from build123d import *
from build123d.topology import SkipClean

# Parameters (mm, degrees)
SKETCH1_R           = 1.2
BOSS_EXTRUDE1_DEPTH = 2.2
BOSS_EXTRUDE2_START = 2.2
SKETCH2_R           = 1.2
BOSS_EXTRUDE2_DEPTH = 2.2
SKETCH3_R           = 1.2
BOSS_EXTRUDE3_DEPTH = 2.2


with BuildPart() as part:
    # Sketch1 → Boss-Extrude1 (new body)
    with BuildSketch(Plane(origin=(0, 0, 0), x_dir=(1, 0, 0), z_dir=(0, 1, 0))):
        with BuildLine():
            Line((-5.035, 1.393945325), (-5.035, 3.24734466))
            Line((-5.035, 3.24734466), (-2.8, 3.24734466))
            Line((-2.8, 3.24734466), (-2.8, 1.393945325))
            ThreePointArc((-2.8, 1.393945325), (-3.9175, -2.24265534), (-5.035, 1.393945325))
        make_face()
        with Locations(Location((-3.9175, -0.25265534, 0), (0, 0, 270))):
            Circle(SKETCH1_R, mode=Mode.SUBTRACT)
    extrude(amount=BOSS_EXTRUDE1_DEPTH)

    # Sketch2 → Boss-Extrude2 (add)
    with SkipClean():  # the faces are left unmerged after this step: merging them gives an invalid solid
        with BuildSketch(Plane.XZ.offset(BOSS_EXTRUDE2_START)):
            Polygon((-3.9175, -3.24734466), (-0.1675, -3.24734466), (-0.1675, 2.75265534), (-7.6675, 2.75265534), (-7.789861557, -3.24734466), align=None)
            with Locations(Location((-3.9175, 0.25265534, 0), (0, 0, 270))):
                Circle(SKETCH2_R, mode=Mode.SUBTRACT)
        extrude(amount=-BOSS_EXTRUDE2_DEPTH)

    # Sketch3 → Boss-Extrude3 (add)
    with BuildSketch(Plane(origin=(0, 2.2, 0), x_dir=(1, 0, 0), z_dir=(0, 1, 0))):
        Polygon((-7.789861557, 3.24734466), (-5.035, 3.24734466), (-2.8, 3.24734466), (-0.1675, 3.24734466), (-0.1675, -2.75265534), (-7.6675, -2.75265534), align=None)
        with Locations(Location((-3.9175, -0.25265534, 0), (0, 0, 90))):
            Circle(SKETCH3_R, mode=Mode.SUBTRACT)
    extrude(amount=BOSS_EXTRUDE3_DEPTH)


solid = part.part
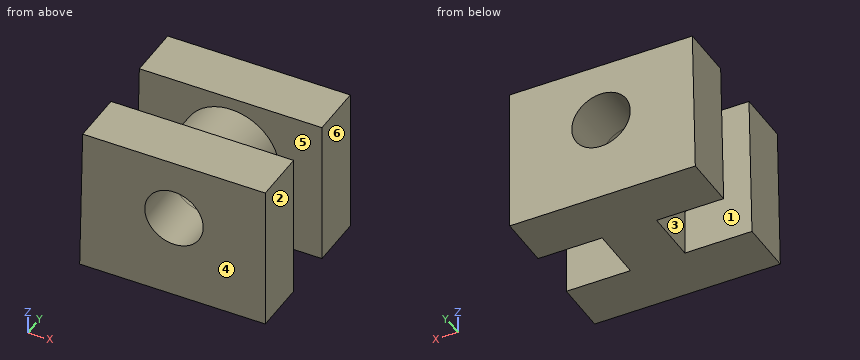
Input: part model. Units: mm. Frame: model coordinates. Face numbers are marked on the shaded views. A direction names the side the tool comes from. Give positions to 0.01 mm unless a question says otherwise; leave off trailing zeros. Order: outer loops, then holes, each group sorted by start corner. A loop starts at its lowest first (then second) coordinate and runs counter-clockwise, first axis right, second up.
Q1. Section B-B on z = -0.85. Output: boundary loops of the cut face in (x, y), and give its area (3 significant figures).
Checked values:
outline: (-7.74, -2.2) - (-4.39, -2.2) - (-4.39, 4.4) - (-7.74, 4.4) - (-7.74, 2.2) - (-5.57, 2.2) - (-5.57, 0) - (-7.74, 0) - close; (-3.44, -2.2) - (-0.17, -2.2) - (-0.17, 0) - (-2.26, 0) - (-2.26, 2.2) - (-0.17, 2.2) - (-0.17, 4.4) - (-3.44, 4.4) - close
area: 34.4 mm2
Q2. Section D-D on y = 3. Output: boundary loops of the cut face in (x, z).
Checked values:
outline: (-7.79, -3.25) - (-0.17, -3.25) - (-0.17, 2.75) - (-7.67, 2.75) - close; hole circle Ø2.4 at (-3.92, 0.25)
Q3. Contact query for a flat-ended pin moving along its axis: pin 1 Ø1.9 at (x, z) = (-3.92, 0.25) entering from +Y. Output: stop coordinate, or through.
Checked values:
pin 1: passes through
Q4. Draft query along Y for the marked faces 4, 5 and 6. Return one class per face: +Y half, -Y half, draft (parallel to the pull), parting line (faces both ways), or undercut.
Checked values:
face 4: -Y half
face 5: undercut
face 6: draft
Q5. Ray query, probe 1 along Y at (x, z) = (-0.5, -1.8); probe 2 along Z at (x, y) = (-3, -0.25); probe 3 along X at (y, z) = (-0.5, 0.3). Return the intervals inside material, ascending.
Checked values:
probe 1: y = -2.2 to 0, 2.2 to 4.4
probe 2: z = -3.25 to -0.52, 1.03 to 2.75
probe 3: x = -7.72 to -5.12, -2.72 to -0.17
Q6. Section A-A on x = -6.25. Output: boundary loops of the cut face in (y, z).
Checked values:
outline: (-2.2, -3.25) - (0, -3.25) - (0, 2.75) - (-2.2, 2.75) - close; (2.2, -3.25) - (4.4, -3.25) - (4.4, 2.75) - (2.2, 2.75) - close
Q7. Section C-C on x = -5.25. Output: boundary loops of the cut face in (y, z).
Checked values:
outline: (-2.2, -3.25) - (0, -3.25) - (0, -1.23) - (2.2, -1.23) - (2.2, -3.25) - (4.4, -3.25) - (4.4, 2.75) - (2.2, 2.75) - (2.2, 1.73) - (0, 1.73) - (0, 2.75) - (-2.2, 2.75) - close
Q8. Set-up query: the marked faces 1, 2 and 3. Return all of +Z, -Z, +X, -X, +Y, -Y with unobstructed straight access to the full face (end or side cutting, diameter ignored); none if empty.
Checked values:
face 1: none
face 2: +Z, -Z, +X, +Y, -Y
face 3: -Z, -X
